Check sheet for the modelled part. Datum: model origin and axes. Units: mm. A direction names the side the tool comes from. Round coordinates to 2 decimals unless told otherwise and drop trailing zeros. Loops run counter-clockwise (first coordinate to the right, second up) from the corner with the lowest first, then second, coordinate; pieces in that order, holes last. Notation, with made-up numbers: (31, 27.25) - (80, 27.25) arc R13 cw to (80, 47.25) - close; hole circle Ø8 at (25.5, -9). An arc over 180 degrees is marked (long way). Return JSON: item names as keys, results as strings.
from build123d import *

# Parameters (mm, degrees)
SKETCH1_R               = 7.5
SKETCH1_R_2             = 0.75
BOSS_EXTRUDE1_DEPTH     = 30
FILLET4_R               = 7.5
SKETCH2_W               = 3.090169944
SKETCH2_H               = 10
BOSS_EXTRUDE2_DEPTH     = 20
SKETCH3_R               = 2
CUT_EXTRUDE1_DEPTH      = 45.300112867
CUT_EXTRUDE4_START      = -45.300113002
SKETCH7_R               = 2
CUT_EXTRUDE4_DEPTH      = 45.400113002
CUT_EXTRUDE5_DEPTH      = 45.300113002
CUT_EXTRUDE5_DEPTH_BACK = 45.300113002
SKETCH7_2_R             = 2
CUT_EXTRUDE8_REACH      = 46.3
SKETCH15_R              = 2.5
BOSS_EXTRUDE3_DEPTH     = 12
SKETCH16_R              = 4
BOSS_EXTRUDE4_DEPTH     = 2
SKETCH13_W              = 1.5
SKETCH13_H              = 8.04181095
CUT_EXTRUDE14_DEPTH     = 48.154003117
SKETCH10_R              = 7.5
CUT_EXTRUDE11_DEPTH     = 28.540878735
REVOLVE1_ANGLE          = 180
SKETCH1_2_R             = 0.75
CUT_EXTRUDE12_DEPTH     = 34.944808167
CUT_EXTRUDE16_DEPTH     = 2


with BuildPart() as part:
    # Sketch1 → Boss-Extrude1 (new body)
    with BuildSketch(Plane(origin=(0, 0, 0), x_dir=(1, 0, 0), z_dir=(0, 1, 0))):
        with Locations(Location((0, 0, 0), (0, 0, 270))):
            Circle(SKETCH1_R)
        with Locations(Location((0, -5, 0), (0, 0, 270))):
            Circle(SKETCH1_R_2, mode=Mode.SUBTRACT)
    extrude(amount=BOSS_EXTRUDE1_DEPTH)

    # Fillet4
    # the kernel refuses this fillet: 7.5 mm, written as the material it takes off along each edge
    with BuildSketch(Plane(origin=(0, 0, 0), x_dir=(0, 0, 1), z_dir=(-1, 0, 0))) as fillet4_piece_1:
        with BuildLine():
            CenterArc((7.5 - FILLET4_R, FILLET4_R), FILLET4_R, 270, 90)
            Line((7.5 - FILLET4_R, 0), (7.5, 0))
            Line((7.5, 0), (7.5, FILLET4_R))
        make_face()
    revolve(axis=Axis((0, 0, 0), (0, 1, 0)), mode=Mode.SUBTRACT)
    with BuildSketch(Plane(origin=(0, 30, 0), x_dir=(0, 0, 1), z_dir=(-1, 0, 0))) as fillet4_piece_2:
        with BuildLine():
            CenterArc((7.5 - FILLET4_R, -FILLET4_R), FILLET4_R, 0, 90)
            Line((7.5 - FILLET4_R, 0), (7.5, 0))
            Line((7.5, 0), (7.5, -FILLET4_R))
        make_face()
    revolve(axis=Axis((0, 30, 0), (0, 1, 0)), mode=Mode.SUBTRACT)

    # Sketch2 → Boss-Extrude2 (add)
    with BuildSketch(Plane(origin=(0, 22.5, 0), x_dir=(1, 0, 0), z_dir=(0, 1, 0))):
        with Locations((4.045084972, 0)):
            Rectangle(SKETCH2_W, SKETCH2_H)
        with BuildLine():
            ThreePointArc((5.590169944, -5), (7.5, 0), (5.590169944, 5))
            Line((5.590169944, 5), (5.590169944, -5))
        make_face()
    boss_extrude2 = extrude(amount=BOSS_EXTRUDE2_DEPTH)

    # Sketch3 → Cut-Extrude1 (cut, symmetric)
    with BuildSketch(Plane.ZY.offset(-2.5)):
        with BuildLine():
            ThreePointArc((-5, 37.5), (-3.535533906, 41.035533906), (0, 42.5))
            Line((0, 42.5), (-5, 42.5))
            Line((-5, 42.5), (-5, 37.5))
        make_face()
        with BuildLine():
            ThreePointArc((0, 42.5), (3.535533906, 41.035533906), (5, 37.5))
            Line((5, 37.5), (5, 42.5))
            Line((5, 42.5), (0, 42.5))
        make_face()
        with Locations(Location((0, 37.5, 0), (0, 0, 270))):
            Circle(SKETCH3_R)
    cut_extrude1 = extrude(amount=CUT_EXTRUDE1_DEPTH, both=True, mode=Mode.SUBTRACT)

    # Sketch7 → Cut-Extrude4 (cut)
    with BuildSketch(Plane.ZY.offset(-2.5).offset(CUT_EXTRUDE4_START)):
        with BuildLine():
            Line((0, 10), (7.5, 10))
            Line((7.5, 10), (7.5, 0))
            Line((7.5, 0), (-5, 0))
            Line((-5, 0), (-5, 5))
            ThreePointArc((-5, 5), (-3.535533906, 8.535533906), (0, 10))
        make_face()
        with Locations(Location((0, 5, 0), (0, 0, 230.136383732))):
            Circle(SKETCH7_R, mode=Mode.SUBTRACT)
    cut_extrude4 = extrude(amount=CUT_EXTRUDE4_DEPTH, mode=Mode.SUBTRACT)

    # Sketch7<2> → Cut-Extrude5 (cut, two sides: drawn at the far end of the back side and taken through both)
    with BuildSketch(Plane.ZY.offset(-2.5).offset(-CUT_EXTRUDE5_DEPTH_BACK)):
        with Locations(Location((0, 5, 0), (0, 0, 222.357273293))):
            Circle(SKETCH7_2_R)
    extrude(amount=CUT_EXTRUDE5_DEPTH + CUT_EXTRUDE5_DEPTH_BACK, mode=Mode.SUBTRACT)

    # Mirror1: Boss-Extrude2, Cut-Extrude1, Cut-Extrude4 across plane
    add(boss_extrude2.mirror(Plane(origin=(0, 0, 0), x_dir=(0, 0, 1), z_dir=(1, 0, 0))))
    add(cut_extrude1.mirror(Plane(origin=(0, 0, 0), x_dir=(0, 0, 1), z_dir=(1, 0, 0))), mode=Mode.SUBTRACT)
    add(cut_extrude4.mirror(Plane(origin=(0, 0, 0), x_dir=(0, 0, 1), z_dir=(1, 0, 0))), mode=Mode.SUBTRACT)

    # Cut-Extrude8: up to this face of the body (flat: up to its plane)
    cut_extrude8_end = Plane(part.part.faces().sort_by_distance((-2.5, 34.956709536, 0))[0])
    # Sketch9 → Cut-Extrude8 (cut, up to the picked face)
    with BuildSketch(Plane.ZY.offset(-2.5), mode=Mode.PRIVATE) as cut_extrude8_sk1:
        with BuildLine():
            Line((5, 27.5), (22.867472592, 27.5))
            Line((22.867472592, 27.5), (22.867472592, 37.5))
            Line((22.867472592, 37.5), (-5, 37.5))
            ThreePointArc((-5, 37.5), (-2.071067812, 30.428932188), (5, 27.5))
        make_face()
    cut_extrude8_tool1 = split(extrude(cut_extrude8_sk1.sketch, amount=CUT_EXTRUDE8_REACH, mode=Mode.PRIVATE), bisect_by=cut_extrude8_end, keep=Keep.BOTH, mode=Mode.PRIVATE)
    add(cut_extrude8_tool1.solids().sort_by(Axis((2.5, 32.730802, 9.909907), (-1, 0, 0)))[0], mode=Mode.SUBTRACT)

    # Sketch15 → Boss-Extrude3 (add)
    with BuildSketch(Plane.XY):
        with Locations((0, 15)):
            Circle(SKETCH15_R)
    extrude(amount=-BOSS_EXTRUDE3_DEPTH)

    # Sketch16 → Boss-Extrude4 (add)
    with BuildSketch(Plane(origin=(0, 0, -12), x_dir=(-1, 0, 0), z_dir=(0, 0, -1))):
        with Locations((0, 15)):
            Circle(SKETCH16_R)
    extrude(amount=BOSS_EXTRUDE4_DEPTH)

    # Sketch13 → Cut-Extrude14 (cut, through all)
    with BuildSketch(Plane.XY.offset(5)):
        with Locations((-1.855e-06, 5.979094525)):
            Rectangle(SKETCH13_W, SKETCH13_H)
    extrude(amount=CUT_EXTRUDE14_DEPTH, mode=Mode.SUBTRACT)

    # Sketch10 → Cut-Extrude11 (cut, through all)
    with BuildSketch(Plane(origin=(0, 22.5, 0), x_dir=(1, 0, 0), z_dir=(0, 1, 0))):
        with Locations(Location((0, 0, 0), (0, 0, 90))):
            Circle(SKETCH10_R)
    extrude(amount=CUT_EXTRUDE11_DEPTH, mode=Mode.SUBTRACT)

    # Sketch11 → Revolve1 (revolve)
    with BuildSketch(Plane(origin=(0, 22.5, 0), x_dir=(1, 0, 0), z_dir=(0, 1, 0))):
        with BuildLine():
            Line((0, 7.5), (0, -7.5))
            ThreePointArc((0, -7.5), (7.5, 0), (0, 7.5))
        make_face()
    revolve(axis=Axis((0, 22.5, -7.5), (0, 0, 1)), revolution_arc=REVOLVE1_ANGLE)

    # Sketch1<2> → Cut-Extrude12 (cut, through all)
    with BuildSketch(Plane(origin=(0, 0, 0), x_dir=(1, 0, 0), z_dir=(0, 1, 0))):
        with Locations(Location((0, -5, 0), (0, 0, 156.648060809))):
            Circle(SKETCH1_2_R)
    extrude(amount=CUT_EXTRUDE12_DEPTH, mode=Mode.SUBTRACT)

    # Sketch14<2> → Cut-Extrude16 (cut, symmetric)
    with BuildSketch(Plane(origin=(0, 0, 0), x_dir=(0, 0, -1), z_dir=(1, 0, 0))):
        Polygon((7.5, 1.909830056), (7.5, 13.090169944), (7.181694991, 15), (5, 1.909830056), align=None)
    extrude(amount=CUT_EXTRUDE16_DEPTH, both=True, mode=Mode.SUBTRACT)


solid = part.part
Q1. Sectioned sample at C-C (z = 3). Enter the section's corners in (x, y), plus the area to 3 significant figures.
Answer key:
{"outline": "(-6.87, 10) - (-2.4, 10) - (-2.4, 1.06) arc R6.87 ccw to (2.4, 1.06) - (2.4, 10) - (6.87, 10) - (6.87, 22.5) arc R6.87 ccw to (-6.87, 22.5) - close", "area": "290 mm²"}
Q2. Sectioned sample at D-D (y = 24). Enter the section's corners in (x, z), plus the area to 3 significant figures.
Answer key:
{"outline": "circle Ø14.7 at (0, 0); hole circle Ø1.5 at (0, 5)", "area": "168 mm²"}
Q3. Tool access check on faces 4 (the face through (4, 10, 3)), 5 (the face through (-4, 8, -4)), 6 (the face through (1.34, 17.11, -9.5)). Record the directions out of +Z, -Z, +X, -X, +Y, -Y that give a thin tool (end or side, any length) a straight path to the whole face; none if there is none.
Answer key:
{"face 4": "+Z, +X, -Y", "face 5": "+Z, -X, -Y", "face 6": "none"}
Q4. Sectioned sample at A-A (x = 0). Enter the section's corners in (y, z), plus the area to 3 significant figures.
Answer key:
{"outline": "(1.32, 4.25) arc R7.5 ccw to (1.91, -5) - (15, -7.18) - (13.09, -7.5) - (12.5, -7.5) - (12.5, -12) - (11, -12) - (11, -14) - (19, -14) - (19, -12) - (17.5, -12) - (17.5, -7.5) - (22.5, -7.5) arc R7.5 ccw to (28.68, 4.25) - close; (10, 5.75) - (27.32, 5.75) arc R7.5 ccw to (22.5, 7.5) - (10, 7.5) - close; hole circle Ø4 at (5, 0)", "area": "364 mm²"}
Q5. Draft check along Z on faces 1 (the face through (3, 4, -5)), 2 (the face through (0.03, 4.32, -1.88)), 3 (the face through (-4, 10, 3)). Enter one of: released by +Z, released by -Z, zero draft, split by the parting line, or undercut.
Answer key:
{"face 1": "released by +Z", "face 2": "undercut", "face 3": "zero draft"}
Q6. Scan lines: probe 1 along X at (y, z) = (3.75, 6); probe 2 along Y at (x, z) = (0.9, 0); probe 3 along X at (y, z) = (14.75, 5.25). Record each from-to range of solid material in increasing order. Write a range as [from, to].
Answer key:
{"probe 1": "x = [-2.4, -0.75], [0.75, 2.4]", "probe 2": "y = [0.05, 3], [7, 29.95]", "probe 3": "x = [-5.36, -0.71], [0.71, 5.36]"}
Q7. Sectioned sample at B-B (y = 12). Enter the section's corners in (x, z), plus the area to 3 significant figures.
Answer key:
{"outline": "(-2.65, -14) - (2.65, -14) - (2.65, -12) - (-2.65, -12) - close; (-2, -7.23) - (-2, -6.68) - (2, -6.68) - (2, -7.23) arc R7.5 ccw (long way) to start; hole circle Ø1.5 at (0, 5)", "area": "183 mm²"}
Q8. Depth check by flat-ended pin: P1, Ø4, axis at x = 5.5, z = 5, coming from the -Y side; P2, Ø2, axis at x = -4, y = 4, coming from the +Z side; P3, Ø3, axis at y = 3.5, z = 0, coming from the +X side. Enter the tip coordinate at first touch or a pass-through.
Answer key:
{"P1": "stops at y = 10", "P2": "stops at z = -5", "P3": "stops at x = 2.4"}
